Read the model definition and answer for the solid it produces. Units are mm, in the model's axes. Face numbers are marked on the shaded views. Round coordinates to 2 decimals unless told otherwise and drop trailing zeros. Order: outer loops, then holes, each group sorted by start corner. A loop starts at its lowest first (then second) coordinate and runs counter-clockwise, first axis right, second up. Notation, with made-up numbers: (-5.75, -33.5) -> (7.25, -33.5) arc R33 cw to (7.25, 2.5) -> close; hole circle Ø6 at (-4.5, 63). An arc over 180 degrees is marked (long way). One line per item, written item: value. Start each with the question number.
1. The mould has two halves that part along Z. Classify the marked faces 1 and 2: released by +Z, released by -Z, zero draft, split by the parting line, or undercut.
2. Section B-B (z = 81.5) is taken. Give the vertices of the cut face in (x, y), then the cut area to 3 significant figures.
3. Consider line 1 (Y direction, x = 182, z = -5); line 2 (Z direction, x = 286, y = 10). Determine where each line is inside the solid, lowest interval first.
4. Section A-A (y = -123) is taken. Give the vertices of the cut face in (x, z).
5. Section D-D (y = -239.5) is taken. Give the vertices of the cut face in (x, z), then the cut area to 3 significant figures.
6. Section C-C (x = 88.5) is taken. Give the vertices of the cut face in (y, z), then the cut area to 3 significant figures.
7. Flat-ended cylindrical pins translate along their axes: pin 1 Ø12.5 at (y, z) = (-152, 337.5) entering from +X; pin 2 Ø7.5 at (x, y) = (302.5, 15.5) entering from +Z; pin 3 Ø12.5 at (y, z) = (-47.5, -176.5) entering from +X. Find the tip coordinate at first contact, or state that the pin passes through.
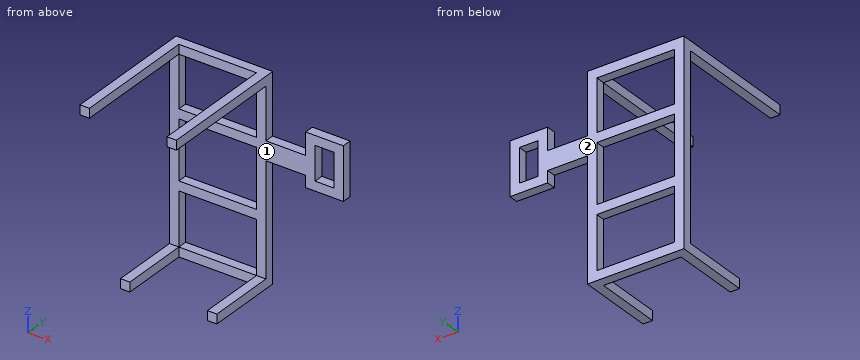
from build123d import *

# Parameters (mm, degrees)
SKETCH2_W           = 260.35
SKETCH2_H           = 209.55
SKETCH2_W_2         = 209.55
SKETCH2_H_2         = 158.75
SKETCH2_W_3         = 50.8
SKETCH2_H_3         = 91.44
SKETCH2_W_4         = 107.2896
SKETCH2_H_4         = 50.8
BOSS_EXTRUDE1_DEPTH = 25.4
SKETCH3_W           = 260.35
SKETCH3_H           = 543.56
SKETCH3_W_2         = 209.55
SKETCH3_H_2         = 492.76
BOSS_EXTRUDE2_DEPTH = 25.4
SKETCH4_W           = 25.4
SKETCH4_H           = 25.4
BOSS_EXTRUDE3_DEPTH = 184.785
SKETCH5_W           = 25.4
SKETCH5_H           = 25.4
BOSS_EXTRUDE4_DEPTH = 337.185


with BuildPart() as part:
    # Sketch2 → Boss-Extrude1 (new body)
    # profile 1 of 3: a face of its own
    with BuildSketch(Plane(origin=(0, 0, 0), x_dir=(1, 0, 0), z_dir=(0, 1, 0))):
        with Locations((104.775, -79.375)):
            Rectangle(SKETCH2_W, SKETCH2_H)
        with Locations((104.775, -79.375)):
            Rectangle(SKETCH2_W_2, SKETCH2_H_2, mode=Mode.SUBTRACT)
    # profile 2 of 3: a face of its own
    with BuildSketch(Plane(origin=(0, 0, 0), x_dir=(1, 0, 0), z_dir=(0, 1, 0))):
        Polygon((342.2396, -133.35), (342.2396, -184.15), (342.2396, -244.094), (443.8396, -244.094), (443.8396, -101.854), (342.2396, -101.854), align=None)
        with Locations((393.0396, -172.974)):
            Rectangle(SKETCH2_W_3, SKETCH2_H_3, mode=Mode.SUBTRACT)
    # profile 3 of 3: a face of its own
    with BuildSketch(Plane(origin=(0, 0, 0), x_dir=(1, 0, 0), z_dir=(0, 1, 0))):
        with Locations((288.5948, -158.75)):
            Rectangle(SKETCH2_W_4, SKETCH2_H_4)
    extrude(amount=BOSS_EXTRUDE1_DEPTH)

    # Sketch3 → Boss-Extrude2 (add)
    with BuildSketch(Plane(origin=(0, 25.4, 0), x_dir=(1, 0, 0), z_dir=(0, 1, 0))):
        with Locations((104.775, -77.47)):
            Rectangle(SKETCH3_W, SKETCH3_H)
        with Locations((104.775, -77.47)):
            Rectangle(SKETCH3_W_2, SKETCH3_H_2, mode=Mode.SUBTRACT)
    extrude(amount=-BOSS_EXTRUDE2_DEPTH)

    # Sketch4 → Boss-Extrude3 (add)
    with BuildSketch(Plane.XZ):
        with Locations((-12.7, -181.61)):
            Rectangle(SKETCH4_W, SKETCH4_H)
        with Locations((222.25, -181.61)):
            Rectangle(SKETCH4_W, SKETCH4_H)
    extrude(amount=BOSS_EXTRUDE3_DEPTH)

    # Sketch5 → Boss-Extrude4 (add)
    with BuildSketch(Plane.XZ):
        with Locations((-12.7, 336.55)):
            Rectangle(SKETCH5_W, SKETCH5_H)
        with Locations((222.25, 336.55)):
            Rectangle(SKETCH5_W, SKETCH5_H)
    extrude(amount=BOSS_EXTRUDE4_DEPTH)


solid = part.part
Answer:
1. face 1: undercut
1. face 2: zero draft
2. outline: (-25.4, 0) -> (0, 0) -> (0, 25.4) -> (-25.4, 25.4) -> close; (209.55, 0) -> (234.95, 0) -> (234.95, 25.4) -> (209.55, 25.4) -> close
2. area: 1,290 mm^2
3. line 1: 0 to 25.4
3. line 2: 133.35 to 184.15
4. outline: (-25.4, -194.31) -> (0, -194.31) -> (0, -168.91) -> (-25.4, -168.91) -> close; (-25.4, 323.85) -> (0, 323.85) -> (0, 349.25) -> (-25.4, 349.25) -> close; (209.55, -194.31) -> (234.95, -194.31) -> (234.95, -168.91) -> (209.55, -168.91) -> close; (209.55, 323.85) -> (234.95, 323.85) -> (234.95, 349.25) -> (209.55, 349.25) -> close
5. outline: (-25.4, 323.85) -> (0, 323.85) -> (0, 349.25) -> (-25.4, 349.25) -> close; (209.55, 323.85) -> (234.95, 323.85) -> (234.95, 349.25) -> (209.55, 349.25) -> close
5. area: 1,290 mm^2
6. outline: (0, -194.31) -> (25.4, -194.31) -> (25.4, -168.91) -> (0, -168.91) -> close; (0, -25.4) -> (25.4, -25.4) -> (25.4, 0) -> (0, 0) -> close; (0, 158.75) -> (25.4, 158.75) -> (25.4, 184.15) -> (0, 184.15) -> close; (0, 323.85) -> (25.4, 323.85) -> (25.4, 349.25) -> (0, 349.25) -> close
6. area: 2,580 mm^2
7. pin 1: x = 234.95
7. pin 2: z = 184.15
7. pin 3: x = 234.95
